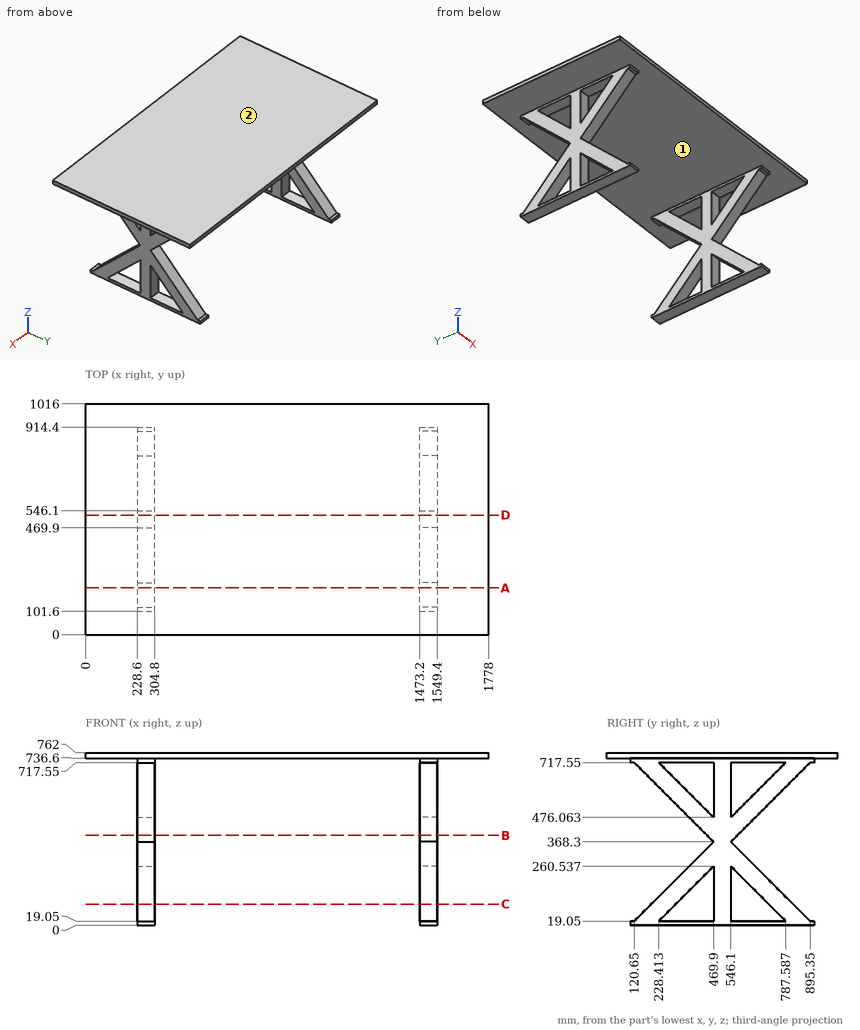
Geometry: see drawing. Coordinates: mm, zero at the bounding-box minimum. Give positions to 0.01 mm unless a question says otherwise; leave off trailing zeros. Write each loop counter-clockwise with the first axis right and the second up, starting at its lowest first coordinate (ties: lowest second). Pieces come first, ordered by that corner, then holes. Notation, with made-up numbers: (75, -7) -> (131, -7) arc R33 ccw to (131, 29) -> close; hole circle Ø6 at (-25.5, 13). An arc over 180 degrees is marked (long way). Use one line per item in the form item = value. Start each with the question number.
1) Pin query (flat end, axial travel): pin 1 (6 mm diameter, centred on x = 1151.5, y = 149, fed in from -Z); pin 2 (15 mm diameter, centred on x = 283.5, z = 9.5, fed in from +Y); pin 3 (1 mm diameter, centred on y = 526, z = 152.5, fed in from +X). Return the tip coordinate at first contact, or that it passes through.
2) Ray query, probe 1 along X at (y, z) = (205.5, 722); probe 2 along Y at (x, z) = (1510, 83); probe 3 along Z at (x, y) = (1344.5, 68). Return the intervals inside material, ascending. Write a range as from..to.
3) Section query D-D on y = 526.5. Return the cut outline in (x, z).
4) Section query A-A on y = 206. Return the cut outline in (x, z), then the cut area to 3 significant figures.
5) Draft query along X for the marked faces 1 and 2. Return one class per face: pulls with the +X half, pulls with the -X half, needs draft (parallel to the pull), parting line crosses it, or undercut.
6) Section query C-C on z = 94. Return the cut outline in (x, y).
7) Section query B-B on z = 397. Return the cut outline in (x, y), then the cut area to 3 significant figures.
Outcome:
q1.pin_1 = 736.6
q1.pin_2 = 914.4
q1.pin_3 = 1549.4
q2.probe_1 = 228.6..304.8, 1473.2..1549.4
q2.probe_2 = 184.6..292.36, 469.9..546.1, 723.64..831.4
q2.probe_3 = 736.6..762
q3.outline = (0, 736.6) -> (228.6, 736.6) -> (228.6, 0) -> (304.8, 0) -> (304.8, 736.6) -> (1473.2, 736.6) -> (1473.2, 0) -> (1549.4, 0) -> (1549.4, 736.6) -> (1778, 736.6) -> (1778, 762) -> (0, 762) -> close
q4.outline = (0, 736.6) -> (228.6, 736.6) -> (228.6, 632.2) -> (304.8, 632.2) -> (304.8, 736.6) -> (1473.2, 736.6) -> (1473.2, 632.2) -> (1549.4, 632.2) -> (1549.4, 736.6) -> (1778, 736.6) -> (1778, 762) -> (0, 762) -> close; (228.6, 0) -> (304.8, 0) -> (304.8, 104.4) -> (228.6, 104.4) -> close; (1473.2, 0) -> (1549.4, 0) -> (1549.4, 104.4) -> (1473.2, 104.4) -> close
q4.area = 77,000 mm^2
q5.face_1 = undercut
q5.face_2 = needs draft
q6.outline = (228.6, 195.6) -> (304.8, 195.6) -> (304.8, 303.36) -> (228.6, 303.36) -> close; (228.6, 469.9) -> (304.8, 469.9) -> (304.8, 546.1) -> (228.6, 546.1) -> close; (228.6, 712.64) -> (304.8, 712.64) -> (304.8, 820.4) -> (228.6, 820.4) -> close; (1473.2, 195.6) -> (1549.4, 195.6) -> (1549.4, 303.36) -> (1473.2, 303.36) -> close; (1473.2, 469.9) -> (1549.4, 469.9) -> (1549.4, 546.1) -> (1473.2, 546.1) -> close; (1473.2, 712.64) -> (1549.4, 712.64) -> (1549.4, 820.4) -> (1473.2, 820.4) -> close
q7.outline = (228.6, 441.2) -> (304.8, 441.2) -> (304.8, 574.8) -> (228.6, 574.8) -> close; (1473.2, 441.2) -> (1549.4, 441.2) -> (1549.4, 574.8) -> (1473.2, 574.8) -> close
q7.area = 20,400 mm^2
